Read the model definition and answer for the solid it produces. Units are mm, in the model's axes. A direction names the side the tool comes from. Give positions to 0.01 mm unless a question says otherwise; leave off trailing zeros. Write each loop counter-clockwise with the first axis right and the second up, starting at its lowest first coordinate (ties: lowest second). Pieces come first, ordered by that corner, then holes. Notation, with made-up numbers: (-18.5, 42.25) -> (-14.5, 42.25) arc R11 ccw to (-14.5, 53.25) -> close; hole circle Ø7 at (-29.5, 19.5). An arc over 180 degrees is marked (long way). Write item = value, one per line.
from build123d import *

# Parameters (mm, degrees)
F1_R     = 2
F2_DEPTH = 3
F3_W     = 7
F3_H     = 15
F4_DEPTH = 7
F5_R     = 2.5
F6_DEPTH = 7
F8_DEPTH = 25


with BuildPart() as f2:
    # F1 (on Top) → F2 (new body)
    with BuildSketch(Plane.XY):
        with BuildLine():
            Line((5.260746949, 48.1550168068), (-1.739253051, 48.1550168068))
            Line((-1.739253051, 48.1550168068), (-1.739253051, 4.1768743183))
            Line((-1.739253051, 4.1768743183), (-17.739253051, 4.1768743183))
            Line((-17.739253051, 4.1768743183), (-17.739253051, -24.0102637737))
            Line((-17.739253051, -24.0102637737), (-10.2988117629, -24.0102637737))
            Line((-10.2988117629, -24.0102637737), (-10.2988117629, -2.8231256817))
            Line((-10.2988117629, -2.8231256817), (8.2878154448, -2.8231256817))
            Line((8.2878154448, -2.8231256817), (8.2878154448, -24.0102637737))
            Line((8.2878154448, -24.0102637737), (13.6364829472, -24.0102637737))
            Line((13.6364829472, -24.0102637737), (13.6364829472, 4.5625712545))
            Line((13.6364829472, 4.5625712545), (5.260746949, 4.5625712545))
            Line((5.260746949, 4.5625712545), (5.260746949, 12.7772765343))
            ThreePointArc((5.260746949, 12.7772765343), (0.6746425074, 14.1550168068), (5.260746949, 15.5327570794))
            Line((5.260746949, 15.5327570794), (5.260746949, 48.1550168068))
        make_face()
        with Locations((-14.0605294946, -19.8449831932)):
            Circle(F1_R, mode=Mode.SUBTRACT)
        with Locations((11.3483034751, -19.8449831932)):
            Circle(F1_R, mode=Mode.SUBTRACT)
    extrude(amount=F2_DEPTH)

    # F3 (on face) → F4 (join)
    with BuildSketch(Plane.XY.offset(3)):
        with Locations((1.760746949, 40.6550168068)):
            Rectangle(F3_W, F3_H)
    extrude(amount=F4_DEPTH)

    # F5 (on face) → F6 (cut, through all)
    with BuildSketch(Plane.YZ.offset(5.260746949)):
        with Locations((40.6550168068, 5)):
            Circle(F5_R)
    extrude(amount=-F6_DEPTH, mode=Mode.SUBTRACT)

    # F7 (on face) → F8 (cut)
    with BuildSketch(Plane.YZ.offset(5.260746949)):
        with BuildLine():
            ThreePointArc((33.1550168068, 7.345077116), (33.9168939811, 8.8286237351), (35.1040102541, 10))
            Line((35.1040102541, 10), (33.1550168068, 10))
            Line((33.1550168068, 10), (33.1550168068, 7.345077116))
        make_face()
        with BuildLine():
            Line((48.1550168068, 10), (46.3816933334, 10))
            ThreePointArc((46.3816933334, 10), (47.6252482208, 8.6215486681), (48.1550168068, 6.8422504701))
            Line((48.1550168068, 6.8422504701), (48.1550168068, 10))
        make_face()
    extrude(amount=-F8_DEPTH, mode=Mode.SUBTRACT)


solid = f2.part
(1) Consider L1, parallel to X at y = -4, z = 2.25; L2, parallel to Y at x = -14, z = 1.75; L3, parallel to Z at x = -4.5, y = 2.5. Determine where each line is inside the solid, lowest interval first.
Checks:
L1 = -17.74 to -10.3, 8.29 to 13.64
L2 = -24.01 to -21.84, -17.85 to 4.18
L3 = 0 to 3
(2) The part is cut by section C-C on y = 32.5. Determine the outline of the cut face in (x, z).
Checks:
outline = (-1.74, 0) -> (5.26, 0) -> (5.26, 3) -> (-1.74, 3) -> close
(3) The part is cut by section A-A on x = 0. Determine the outline of the cut face in (y, z), plus the area to 3 significant figures.
Checks:
outline = (-2.82, 0) -> (48.16, 0) -> (48.16, 6.84) arc R4.21 ccw to (46.38, 10) -> (35.1, 10) arc R5.27 ccw to (33.16, 7.35) -> (33.16, 3) -> (-2.82, 3) -> close; hole circle Ø5 at (40.66, 5)
area = 234 mm²
(4) Given P1, Ø2.5, axis at x = -12.5, z = 2, coming from the +Y side; P2, Ø3, axis at y = 32.5, z = 5.5, coming from the +X side; P3, Ø1.3, axis at x = 2.5, z = 6, coming from the -Y side (3 decimals), each flat-ended and moving along its own axis, determine where each tip first touches the part or whether it passes through.
Checks:
P1 = 4.18
P2 = 5.26
P3 = 33.155
(5) A tool of negligible diameter and unlimited length cuts with its end or side. For faces 1 (the flat face through (-1, 0, 3)), 2 (the flat face through (-1.739, 30.7, 2.7)), 3 (the flat face through (5.261, 9, 1)), from which of +Z, -Z, +X, -X, +Y, -Y can it reach the whole face along a straight path? Write none if from no direction.
Checks:
face_1 = +Z, +X, -X, -Y
face_2 = +Z, -Z, -X, +Y
face_3 = +Z, -Z, +X, +Y
(6) The part is cut by section B-B on z = 1.5. Determine the outline of the cut face in (x, y).
Checks:
outline = (-17.74, -24.01) -> (-10.3, -24.01) -> (-10.3, -2.82) -> (8.29, -2.82) -> (8.29, -24.01) -> (13.64, -24.01) -> (13.64, 4.56) -> (5.26, 4.56) -> (5.26, 12.78) arc R2.5 cw (long way) to (5.26, 15.53) -> (5.26, 48.16) -> (-1.74, 48.16) -> (-1.74, 4.18) -> (-17.74, 4.18) -> close; hole circle Ø4 at (-14.06, -19.84); hole circle Ø4 at (11.35, -19.84)
(7) For a pull along X with two mould halves and no side action, classify faces 4 (the flat face through (-17.739, -10, 1)), 5 (the flat face through (5.261, 35, 4)), 6 (the flat face through (10, 4.563, 1)), 7 (the flat face through (-1, -2.823, 1)) as released by +X, released by -X, zero draft, split by the parting line, or undercut.
Checks:
face_4 = released by -X
face_5 = released by +X
face_6 = zero draft
face_7 = undercut
(8) The part is cut by section D-D on x = 10. Determine the outline of the cut face in (y, z).
Checks:
outline = (-24.01, 0) -> (-21.32, 0) -> (-21.32, 3) -> (-24.01, 3) -> close; (-18.37, 0) -> (4.56, 0) -> (4.56, 3) -> (-18.37, 3) -> close
